```python
from build123d import *

# Parameters (mm, degrees)
F0_W     = 45
F0_H     = 45
F0_R     = 2
F0_R_2   = 18.55
F1_DEPTH = 22.5
F0_R_3   = 17.05
F2_DEPTH = 15.5
F0_R_4   = 12.5
F4_DEPTH = 15
F5_START = -15
F3_R     = 10.825
F5_DEPTH = 30
F6_START = 15
F6_DEPTH = 30
F8_START = 15
F7_R     = 10.825
F8_DEPTH = 10
F9_START = -15
F9_DEPTH = 10


with BuildPart() as f1:
    # F0 (on Front) → F1 (new body, symmetric)
    with BuildSketch(Plane.XZ):
        Rectangle(F0_W, F0_H)
        with Locations((-17.5, -17.5)):
            Circle(F0_R, mode=Mode.SUBTRACT)
        with Locations((17.5, -17.5)):
            Circle(F0_R, mode=Mode.SUBTRACT)
        with Locations((-17.5, 17.5)):
            Circle(F0_R, mode=Mode.SUBTRACT)
        Circle(F0_R_2, mode=Mode.SUBTRACT)
        with Locations((17.5, 17.5)):
            Circle(F0_R, mode=Mode.SUBTRACT)
        with Locations((-17.5, 17.5)):
            Circle(F0_R)
        with Locations((17.5, 17.5)):
            Circle(F0_R)
        with Locations((17.5, -17.5)):
            Circle(F0_R)
        with Locations((-17.5, -17.5)):
            Circle(F0_R)
    extrude(amount=F1_DEPTH, both=True)

    # F0 (on Front) → F2 (join, symmetric)
    with BuildSketch(Plane.XZ):
        Circle(F0_R_2)
        Circle(F0_R_3, mode=Mode.SUBTRACT)
    extrude(amount=F2_DEPTH, both=True)

    # F0 (on Front) → F4 (join, symmetric)
    with BuildSketch(Plane.XZ):
        Circle(F0_R_3)
        Circle(F0_R_4, mode=Mode.SUBTRACT)
    extrude(amount=F4_DEPTH, both=True)

    # F3 (on Right) → F5 (cut)
    with BuildSketch(Plane.YZ.offset(F5_START)):
        Circle(F3_R)
    extrude(amount=-F5_DEPTH, mode=Mode.SUBTRACT)

    # F3 (on Right) → F6 (cut)
    with BuildSketch(Plane.YZ.offset(F6_START)):
        Circle(F3_R)
    extrude(amount=F6_DEPTH, mode=Mode.SUBTRACT)

    # F7 (on Top) → F8 (cut)
    with BuildSketch(Plane.XY.offset(F8_START)):
        Circle(F7_R)
    extrude(amount=F8_DEPTH, mode=Mode.SUBTRACT)

    # F7 (on Top) → F9 (cut)
    with BuildSketch(Plane.XY.offset(F9_START)):
        Circle(F7_R)
    extrude(amount=-F9_DEPTH, mode=Mode.SUBTRACT)


solid = f1.part
```
Geometry check sheet. Reference: the model listing, model coordinates, mm. A direction names the side the tool comes from. Give positions to 0.01 mm unless a question says otherwise; leave off trailing zeros. Write each loop counter-clockwise with the first axis right and the second up, starting at its lowest first coordinate (ties: lowest second). Pieces come first, ordered by that corner, then holes. Notation, with made-up numbers: (-14.5, -39.5) -> (19.5, -39.5) arc R30 ccw to (19.5, -0.5) -> close; hole circle Ø5 at (-27, 11.5). An arc over 180 degrees is marked (long way). One line per question, with ' | ' between items.
Item 1: Sectioned sample at D-D, the plane x = -14. Record the boundary of the cut face in (y, z), plus the area to 3 significant figures.
Determined:
outline: (-22.5, -22.5) -> (22.5, -22.5) -> (22.5, -12.17) -> (15.5, -12.17) -> (15.5, -9.73) -> (15, -9.73) -> (15, 9.73) -> (15.5, 9.73) -> (15.5, 12.17) -> (22.5, 12.17) -> (22.5, 22.5) -> (-22.5, 22.5) -> (-22.5, 12.17) -> (-15.5, 12.17) -> (-15.5, 9.73) -> (-15, 9.73) -> (-15, -9.73) -> (-15.5, -9.73) -> (-15.5, -12.17) -> (-22.5, -12.17) -> close | area: 1,660 mm^2
Item 2: Scan lines: line 1 along Z through (x, y) = (0, 4.25); line 2 along Z through (x, y) = (0, 15.35); line 3 along Y through (x, z) = (-13.5, -4). Record each from-to range of solid material in increasing order.
Determined:
line 1: -15 to -12.5, 12.5 to 15 | line 2: -22.5 to -17.05, 17.05 to 22.5 | line 3: -15 to 15
Item 3: Draft check along Y on faces 5 (the cylindrical face through (-8.59, -6.59, -18.7)), 6 (the cylindrical face through (-2.415, 19.049, 18.392)), 7 (the flat face through (16.4, -15.5, -5.4)). Enter one of: released by +Y, released by -Y, zero draft, split by the parting line, or undercut.
Determined:
face 5: undercut | face 6: zero draft | face 7: released by -Y
Item 4: Sectioned sample at C-C, the plane y = 0. Record the boundary of the cut face in (x, z) (3 decimals).
Determined:
outline: (-22.5, -22.5) -> (-10.825, -22.5) -> (-10.825, -15) -> (10.825, -15) -> (10.825, -22.5) -> (22.5, -22.5) -> (22.5, -10.825) -> (15, -10.825) -> (15, 10.825) -> (22.5, 10.825) -> (22.5, 22.5) -> (10.825, 22.5) -> (10.825, 15) -> (-10.825, 15) -> (-10.825, 22.5) -> (-22.5, 22.5) -> (-22.5, 10.825) -> (-15, 10.825) -> (-15, -10.825) -> (-22.5, -10.825) -> close; hole circle Ø25 at (0, 0)
Item 5: Access from +Z, -Z, +X, -X, +Y, -Y to the whole of each face (thin tool, end or side, straight path). Record for faces 1 (the cylindrical face through (18.7, -8.59, -6.59)), 2 (the flat face through (-15, 0, 0)), 3 (the flat face through (-9, -15, 9)), 4 (the flat face through (-9, 15, 9)).
Determined:
face 1: +X | face 2: -X | face 3: -Y | face 4: +Y
Item 6: Depth check by flat-ended pin: pin 1 (17.5 mm diameter, centred on x = -4, y = -3.5, fed in from +Z); pin 2 (13 mm diameter, centred on x = 0, y = 0, fed in from +Z); pin 3 (11 mm diameter, centred on y = -1.5, z = 1.5, fed in from -X); pin 4 (3 mm diameter, centred on x = 13, z = -7.5, fed in from +Y). Enter the tip coordinate at first touch or a pass-through.
Determined:
pin 1: z = 22.5 | pin 2: z = 15 | pin 3: x = -15 | pin 4: y = 15
